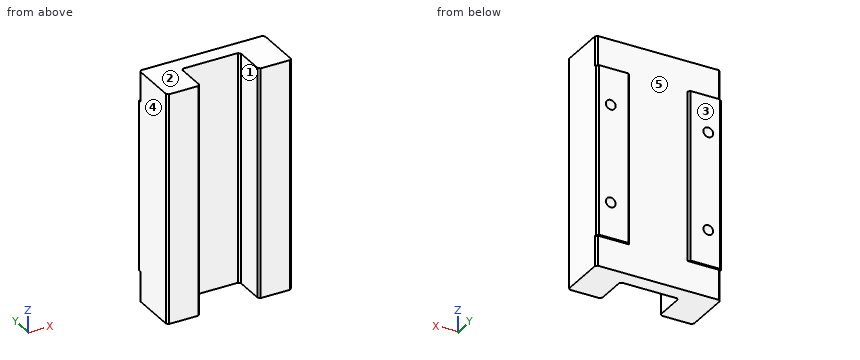
from build123d import *

# Parameters (mm, degrees)
SKETCH1_W                 = 32
SKETCH1_H                 = 43.4
SKETCH1_H_2               = 7.7
BOSS_EXTRUDE1_DEPTH       = 13
M3X0_5_TAPPED_HOLE1_D     = 2.5
M3X0_5_TAPPED_HOLE1_DEPTH = 6.5
M3X0_5_TAPPED_HOLE1_TIP   = 0.751075774
CUT_EXTRUDE1_DEPTH        = 69.194134645
SKETCH5_W                 = 15
SKETCH5_H                 = 43.4
CUT_EXTRUDE2_DEPTH        = 0.5
CHAMFER1_SIZE             = 0.5


with BuildPart() as part:
    # Sketch1 → Boss-Extrude1 (new body)
    with BuildSketch(Plane(origin=(0, 0, 0), x_dir=(1, 0, 0), z_dir=(0, 1, 0))):
        with Locations((16, 29.4)):
            Rectangle(SKETCH1_W, SKETCH1_H)
        with Locations((16, 3.85)):
            Rectangle(SKETCH1_W, SKETCH1_H_2)
        with Locations((16, 54.95)):
            Rectangle(SKETCH1_W, SKETCH1_H_2)
    extrude(amount=BOSS_EXTRUDE1_DEPTH)

    # M3x0.5 Tapped Hole1
    with Locations(Plane(origin=(0, 13, 0), x_dir=(1, 0, 0), z_dir=(0, 1, 0))):
        with Locations((28.5, 17), (28.5, 42), (3.5, 42), (3.5, 17)):
            Hole(M3X0_5_TAPPED_HOLE1_D / 2, depth=M3X0_5_TAPPED_HOLE1_DEPTH)
            with Locations((0, 0, -(M3X0_5_TAPPED_HOLE1_DEPTH + M3X0_5_TAPPED_HOLE1_TIP / 2))):  # 118° drill point
                Cone(0, M3X0_5_TAPPED_HOLE1_D / 2, M3X0_5_TAPPED_HOLE1_TIP, mode=Mode.SUBTRACT)

    # Sketch4 → Cut-Extrude1 (cut, through all)
    with BuildSketch(Plane.XY):
        Polygon((8.5, 8.5), (8.5, 0), (23.5, 0), (23.5, 8.5), (16, 8.5), align=None)
    extrude(amount=-CUT_EXTRUDE1_DEPTH, mode=Mode.SUBTRACT)

    # Sketch5 → Cut-Extrude2 (cut)
    with BuildSketch(Plane(origin=(0, 13, 0), x_dir=(1, 0, 0), z_dir=(0, 1, 0))):
        Polygon((0, 58.8), (0, 51.1), (8.5, 51.1), (23.5, 51.1), (32, 51.1), (32, 58.8), align=None)
        Polygon((8.5, 7.7), (0, 7.7), (0, 0), (32, 0), (32, 7.7), (23.5, 7.7), align=None)
        with Locations((16, 29.4)):
            Rectangle(SKETCH5_W, SKETCH5_H)
    extrude(amount=-CUT_EXTRUDE2_DEPTH, mode=Mode.SUBTRACT)

    # Chamfer1
    chamfer1_edges = [part.edges().sort_by_distance(p)[0] for p in [
        (0, 13, -29.4),
        (8.5, 13, -29.4),
        (0, 12.5, -3.85),
        (0, 12.5, -54.95),
        (0, 0, -29.4),
        (32, 12.5, -3.85),
        (32, 12.5, -54.95),
        (8.5, 0, -29.4),
        (8.5, 8.5, -29.4),
        (23.5, 8.5, -29.4),
        (23.5, 0, -29.4),
        (32, 0, -29.4),
        (32, 13, -29.4),
        (23.5, 13, -29.4),
    ]]
    chamfer(chamfer1_edges, length=CHAMFER1_SIZE - 0.0001)  # a hair under: the kernel refuses the full size


solid = part.part
Geometry: final body of the model. Coordinates: model frame, mm. Face numbers are marked on the shaded views. A direction names the side the tool comes from. Round coordinates to 2 decimals unless told otherwise and drop trailing zeros. Order: outer loops, then holes, each group sorted by start corner. A loop starts at its lowest first (then second) coordinate and runs counter-clockwise, first axis right, second up. Notation, with made-up numbers: (74.25, 81.5) -> (104.25, 81.5) arc R19 cw to (104.25, 86.5) -> close; hole circle Ø11 at (33.5, 0.5). An arc over 180 degrees is marked (long way). Put each result on its own line as item: value. Start each with the question number.
Q1. Pull-direction query (X, two-part tool) for the marked faces 3, 4 and 5; classes: +X half, -X half, draft (parallel to the pull), parting line (faces both ways), or undercut.
Q2. Section A-A on y = 3.75. Return the cut outline in (x, z).
Q3. Section C-C on x = 16.5. Return the cut outline in (y, z), and give its area (3 significant figures).
Q4. First-contact query: pin 1 (2 mm diameter, centred on x = 3.5, z = -17, fed in from +Y); pin 2 (3 mm diameter, centred on x = 15.5, z = -48.5, fed in from -Y). Flat tips, straight axial feed; report the tip coordinate or a pass-through.
Q5. Line query: probe 1 along Z at (x, y) = (3.5, 9.5); probe 2 along X at (y, z) = (9.5, -17); probe 3 along X at (y, z) = (2, -14.5). Output: solid intervals per line, ascending.
Q6. Reachability of the marked faces 1 and 2 from +Z, -Z, +X, -X, +Y, -Y: full face, straight path, thin tool, end or side. Return the list, or none.
Q7. Section D-D on z = -7. Return the cut outline in (x, y).
Ans:
1. face 3: draft
1. face 4: -X half
1. face 5: undercut
2. outline: (0, -58.8) -> (8.5, -58.8) -> (8.5, 0) -> (0, 0) -> close; (23.5, -58.8) -> (32, -58.8) -> (32, 0) -> (23.5, 0) -> close
3. outline: (8.5, -58.8) -> (12.5, -58.8) -> (12.5, 0) -> (8.5, 0) -> close
3. area: 235 mm2
4. pin 1: stops at y = 6.35
4. pin 2: stops at y = 8.5
5. probe 1: z = -58.8 to -43.25, -40.75 to -18.25, -15.75 to 0
5. probe 2: x = 0 to 2.25, 4.75 to 27.25, 29.75 to 32
5. probe 3: x = 0 to 8.5, 23.5 to 32
6. face 1: +Z, -Z, -Y
6. face 2: +Z, +X, -X, +Y, -Y
7. outline: (0, 0.5) -> (0.5, 0) -> (8, 0) -> (8.5, 0.5) -> (8.5, 8) -> (9, 8.5) -> (23, 8.5) -> (23.5, 8) -> (23.5, 0.5) -> (24, 0) -> (31.5, 0) -> (32, 0.5) -> (32, 12) -> (31.5, 12.5) -> (0.5, 12.5) -> (0, 12) -> close
